Check sheet for the modelled part. Datum: model origin and axes. Units: mm. Face numbers are marked on the shaded views. A direction names the side the tool comes from. Coordinates: 2 decimals unless noted, no trailing zeros. Write each loop counter-clockwise with the first axis right and the second up, starting at its lowest first coordinate (ties: lowest second). Pieces come first, ordered by that corner, then holes. Notation, with made-up numbers: (34, 57.25) - (71, 57.25) arc R20 cw to (71, 84.25) - close; hole circle Ø11 at (-31, 87). An arc over 180 degrees is marked (long way). Use one line per item in the form item = value. Start each with the question number.
1. Cross-section at B-B on x = -8.5. Record the boundary of the cut face in (y, z), then the cut area to 3 significant figures.
2. Tool access check on the marked faces 4, 5 and 6. Record the directions out of +Z, -Z, +X, -X, +Y, -Y that give a thin tool (end or side, any length) a straight path to the whole face; none if there is none.
3. Cross-section at A-A on y = 38. Record the boundary of the cut face in (x, z).
4. Scan lines: line 1 along Z through (x, y) = (7.75, 53); line 2 along Y through (x, z) = (10, 24.5); line 3 along Y through (x, z) = (8.5, 8). Record each from-to range of solid material in increasing order.
5. Draft check along Y on the marked faces 1, 2 and 3. Enter one of: +Y half, -Y half, draft (parallel to the pull), parting line (faces both ways), or undercut.
6. Cross-section at C-C on x = 8. Record the boundary of the cut face in (y, z).
7. Go/stop test with flat-tipped pins: pin 1 Ø3.5 at (y, z) = (68, 32) entering from -X; pin 2 Ø8.5 at (x, z) = (0.5, 23) entering from -Y; pin 3 Ø3.5 at (y, z) = (0.5, 16) entering from -X. Record where each tip stops, or that it passes through.
8. Cross-section at D-D on y = 24.5. Record the boundary of the cut face in (x, z).
```python
from build123d import *

# Parameters (mm, degrees)
BOSS_EXTRUDE1_DEPTH = 56
CUT_EXTRUDE1_DEPTH  = 56
CUT_EXTRUDE2_DEPTH  = 10


with BuildPart() as part:
    # Sketch1 → Boss-Extrude1 (new body)
    with BuildSketch(Plane.XY):
        with BuildLine():
            Line((13.02, -7.9417418), (17.7, -7.9417418))
            Line((17.7, -7.9417418), (17.7, 70.02))
            Line((17.7, 70.02), (-10.566443095, 70.02))
            Line((-10.566443095, 70.02), (-10.566443095, 13.02))
            Line((-10.566443095, 13.02), (-5.317126718, 13.02))
            Line((-5.317126718, 13.02), (-4.287512407, 13.02))
            ThreePointArc((-4.287512407, 13.02), (-3.319474451, 12.619025549), (-2.9185, 11.650987593))
            Line((-2.9185, 11.650987593), (-2.9185, 11.539212407))
            ThreePointArc((-2.9185, 11.539212407), (-3.319474451, 10.571174451), (-4.287512407, 10.1702))
            Line((-4.287512407, 10.1702), (-6.476788598, 10.1702))
            ThreePointArc((-6.476788598, 10.1702), (-7.136510935, 9.729114651), (-6.981020848, 8.950903446))
            Line((-6.981020848, 8.950903446), (-3.672257405, 5.649701928))
            ThreePointArc((-3.672257405, 5.649701928), (-2.746830644, 5.032499411), (-1.655778399, 4.8158))
            Line((-1.655778399, 4.8158), (1.655778399, 4.8158))
            ThreePointArc((1.655778399, 4.8158), (2.746830644, 5.032499411), (3.672257405, 5.649701928))
            Line((3.672257405, 5.649701928), (6.981020848, 8.950903446))
            ThreePointArc((6.981020848, 8.950903446), (7.136510935, 9.729114651), (6.476788598, 10.1702))
            Line((6.476788598, 10.1702), (4.287512407, 10.1702))
            ThreePointArc((4.287512407, 10.1702), (3.319474451, 10.571174451), (2.9185, 11.539212407))
            Line((2.9185, 11.539212407), (2.9185, 11.650987593))
            ThreePointArc((2.9185, 11.650987593), (3.319474451, 12.619025549), (4.287512407, 13.02))
            Line((4.287512407, 13.02), (6.332886163, 13.02))
            Line((6.332886163, 13.02), (10.562594215, 13.019824354))
            ThreePointArc((10.562594215, 13.019824354), (12.303594776, 12.313982883), (13.019956614, 10.577284622))
            Line((13.019956614, 10.577284622), (13.02, 4.287469289))
            ThreePointArc((13.02, 4.287469289), (12.619025549, 3.319431332), (11.650987593, 2.918456882))
            Line((11.650987593, 2.918456882), (11.539212407, 2.918456882))
            ThreePointArc((11.539212407, 2.918456882), (10.571174451, 3.319431332), (10.1702, 4.287469289))
            Line((10.1702, 4.287469289), (10.1702, 6.402089023))
            ThreePointArc((10.1702, 6.402089023), (9.733877283, 7.055496588), (8.963146507, 6.90287605))
            Line((8.963146507, 6.90287605), (5.667020993, 3.614283579))
            ThreePointArc((5.667020993, 3.614283579), (5.046449321, 2.687255303), (4.8285, 1.593185507))
            Line((4.8285, 1.593185507), (4.8285, -1.593185507))
            ThreePointArc((4.8285, -1.593185507), (5.046449321, -2.687255303), (5.667020993, -3.614283579))
            Line((5.667020993, -3.614283579), (8.963146507, -6.90287605))
            ThreePointArc((8.963146507, -6.90287605), (9.733877283, -7.055496588), (10.1702, -6.402089023))
            Line((10.1702, -6.402089023), (10.1702, -4.287469289))
            ThreePointArc((10.1702, -4.287469289), (10.571174451, -3.319431332), (11.539212407, -2.918456882))
            Line((11.539212407, -2.918456882), (11.650987593, -2.918456882))
            ThreePointArc((11.650987593, -2.918456882), (12.619025549, -3.319431332), (13.02, -4.287469289))
            Line((13.02, -4.287469289), (13.02, -5.3170836))
            Line((13.02, -5.3170836), (13.02, -7.9417418))
        make_face()
    extrude(amount=BOSS_EXTRUDE1_DEPTH)

    # Sketch14 → Cut-Extrude1 (cut)
    with BuildSketch(Plane(origin=(17.7, 0, 0), x_dir=(0, 0, -1), z_dir=(1, 0, 0))):
        Polygon((-43.675189669, 21.02), (-12.675189669, 21.02), (-7, 26.695189669), (-7, 57.695189669), (-12.324810331, 63.02), (-43.324810331, 63.02), (-49, 57.344810331), (-49, 26.344810331), align=None)
    extrude(amount=-CUT_EXTRUDE1_DEPTH, mode=Mode.SUBTRACT)

    # Sketch15 → Cut-Extrude2 (cut)
    with BuildSketch(Plane(origin=(0, 70.02, 0), x_dir=(1, 0, 0), z_dir=(0, 1, 0))):
        Polygon((-10.566443095, -19), (1.433556905, -19), (1.433556905, -37), (-10.566443095, -37), (-15.100276482, -37), (-15.100276482, -19), align=None)
    extrude(amount=-CUT_EXTRUDE2_DEPTH, mode=Mode.SUBTRACT)


solid = part.part
```
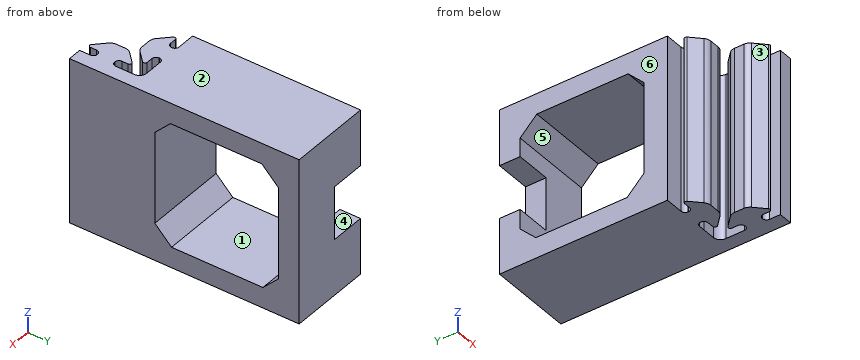
Final values:
q1.outline = (13.02, 0) - (70.02, 0) - (70.02, 19) - (63.02, 19) - (63.02, 12.32) - (57.7, 7) - (26.7, 7) - (21.02, 12.68) - (21.02, 43.68) - (26.34, 49) - (57.34, 49) - (63.02, 43.32) - (63.02, 37) - (70.02, 37) - (70.02, 56) - (13.02, 56) - close
q1.area = 1,360 mm²
q2.face_4 = -X, +Y
q2.face_5 = +X, -X
q2.face_6 = +Z, -Z, -X, +Y, -Y
q3.outline = (-10.57, 0) - (17.7, 0) - (17.7, 7) - (-10.57, 7) - close; (-10.57, 49) - (17.7, 49) - (17.7, 56) - (-10.57, 56) - close
q4.line_1 = 0 to 7, 49 to 56
q4.line_2 = -6.86 to 6.86, 13.02 to 21.02, 63.02 to 70.02
q4.line_3 = -6.44 to 6.44, 13.02 to 25.7, 58.7 to 70.02
q5.face_1 = undercut
q5.face_2 = draft
q5.face_3 = -Y half
q6.outline = (-5.94, 0) - (5.94, 0) - (5.94, 56) - (-5.94, 56) - close; (13.02, 0) - (70.02, 0) - (70.02, 56) - (13.02, 56) - close; hole (21.02, 12.68) - (26.7, 7) - (57.7, 7) - (63.02, 12.32) - (63.02, 43.32) - (57.34, 49) - (26.34, 49) - (21.02, 43.68) - close
q7.pin_1 = 1.43
q7.pin_2 = 4.82
q7.pin_3 = 4.83
q8.outline = (-10.57, 0) - (17.7, 0) - (17.7, 9.2) - (-10.57, 9.2) - close; (-10.57, 47.16) - (17.7, 47.16) - (17.7, 56) - (-10.57, 56) - close
